Design review of the part built by this model. Coordinates are the model's own, in mm. A direction names the side the tool comes from. Round coordinates to 2 decimals unless told otherwise and drop trailing zeros. Order: outer loops, then holes, each group sorted by start corner. A loop starts at its lowest first (then second) coordinate and runs counter-clockwise, first axis right, second up. Notation, with made-up numbers: (34, -26.5) - (49, -26.5) arc R26 ccw to (49, -0.5) - close; hole circle Ø2 at (28.25, 87). An arc over 180 degrees is marked (long way). Write item = value, one per line.
from build123d import *

# Parameters (mm, degrees)
BOSS_EXTRUDE4_DEPTH = 3
FILLET1_R           = 0.5


with BuildPart() as part:
    # Sketch1 → Boss-Extrude4 (new body)
    with BuildSketch(Plane(origin=(0, 0, 0), x_dir=(1, 0, 0), z_dir=(0, 1, 0))):
        Polygon((-369.811676083, 283.948122897), (-399.811676083, 283.948122897), (-399.811676083, 243.948122897), (-319.811676083, 243.948122897), (-319.811676083, 283.948122897), (-349.811676083, 283.948122897), (-354.811676083, 283.948122897), (-354.811676083, 278.948122897), (-324.811676083, 278.948122897), (-324.811676083, 248.948122897), (-394.811676083, 248.948122897), (-394.811676083, 278.948122897), (-364.811676083, 278.948122897), (-364.811676083, 283.948122897), align=None)
        Polygon((-369.811676083, 293.948122897), (-369.811676083, 283.948122897), (-364.811676083, 283.948122897), (-364.811676083, 288.948122897), (-354.811676083, 288.948122897), (-354.811676083, 283.948122897), (-349.811676083, 283.948122897), (-349.811676083, 293.948122897), align=None)
    extrude(amount=BOSS_EXTRUDE4_DEPTH)

    # Fillet1
    fillet1_edges = [part.edges().sort_by_distance(p)[0] for p in [
        (-349.811676083, 3, -288.948122897),
        (-359.811676083, 3, -293.948122897),
        (-364.811676083, 0, -283.948122897),
        (-379.811676083, 0, -278.948122897),
        (-394.811676083, 0, -263.948122897),
        (-369.811676083, 3, -288.948122897),
        (-359.811676083, 0, -248.948122897),
        (-324.811676083, 0, -263.948122897),
        (-339.811676083, 0, -278.948122897),
        (-354.811676083, 0, -283.948122897),
        (-359.811676083, 0, -288.948122897),
        (-319.811676083, 0, -263.948122897),
        (-359.811676083, 0, -243.948122897),
        (-384.811676083, 3, -283.948122897),
        (-349.811676083, 0, -288.948122897),
        (-334.811676083, 0, -283.948122897),
        (-399.811676083, 3, -263.948122897),
        (-364.811676083, 1.5, -288.948122897),
        (-364.811676083, 1.5, -278.948122897),
        (-394.811676083, 1.5, -278.948122897),
        (-359.811676083, 3, -243.948122897),
        (-394.811676083, 1.5, -248.948122897),
        (-324.811676083, 1.5, -278.948122897),
        (-354.811676083, 1.5, -278.948122897),
        (-354.811676083, 1.5, -288.948122897),
        (-319.811676083, 1.5, -283.948122897),
        (-319.811676083, 1.5, -243.948122897),
        (-399.811676083, 1.5, -243.948122897),
        (-349.811676083, 1.5, -293.948122897),
        (-349.811676083, 1.5, -283.948122897),
        (-319.811676083, 3, -263.948122897),
        (-359.811676083, 3, -288.948122897),
        (-354.811676083, 3, -283.948122897),
        (-339.811676083, 3, -278.948122897),
        (-334.811676083, 3, -283.948122897),
        (-324.811676083, 3, -263.948122897),
        (-359.811676083, 3, -248.948122897),
        (-394.811676083, 3, -263.948122897),
        (-379.811676083, 3, -278.948122897),
        (-364.811676083, 3, -283.948122897),
    ]]
    fillet(fillet1_edges, radius=FILLET1_R)


solid = part.part
1) To check wall thickness, follow L1, parallel to X at y = 2.1, z = -263; L2, parallel to Z at x = -387, y = 1.8; L3, parallel to X at y = 2.6, z = -287.5. State the ranges of each line that lie inside material, in increasing order. Write a range as from..to.
Findings:
L1 = -399.81..-394.81, -324.81..-319.81
L2 = -283.95..-278.95, -248.95..-243.95
L3 = -369.8..-364.82, -354.8..-349.82
2) Clearance check with flat-ended pins moving along their axes: pin 1 Ø1.6 at (x, y) = (-329.5, 2) entering from -Z; pin 2 Ø0.6 at (y, z) = (2, -289) entering from +X; pin 3 Ø2 at (x, z) = (-368.5, -277) entering from -Y; pin 4 Ø0.8 at (y, z) = (2, -288) entering from -X. State where each tip first meets the part, or that it passes through.
Findings:
pin_1 = -283.95
pin_2 = -349.81
pin_3 = through
pin_4 = -369.81
3) We need section B-B on x = -352.5. Write out the cut boundary in (y, z), and give its area (3 significant figures).
Findings:
outline = (0, -293.95) - (2.5, -293.95) arc R0.5 ccw to (3, -293.45) - (3, -279.45) arc R0.5 ccw to (2.5, -278.95) - (0.5, -278.95) arc R0.5 ccw to (0, -279.45) - close; (0, -248.45) arc R0.5 ccw to (0.5, -248.95) - (2.5, -248.95) arc R0.5 ccw to (3, -248.45) - (3, -244.45) arc R0.5 ccw to (2.5, -243.95) - (0.5, -243.95) arc R0.5 ccw to (0, -244.45) - close
area = 59.6 mm^2
4) We need section A-A on z = -272.5. Write out the cut boundary in (x, y).
Findings:
outline = (-399.81, 0) - (-395.31, 0) arc R0.5 ccw to (-394.81, 0.5) - (-394.81, 2.5) arc R0.5 ccw to (-395.31, 3) - (-399.31, 3) arc R0.5 ccw to (-399.81, 2.5) - close; (-324.81, 0.5) arc R0.5 ccw to (-324.31, 0) - (-320.31, 0) arc R0.5 ccw to (-319.81, 0.5) - (-319.81, 2.5) arc R0.5 ccw to (-320.31, 3) - (-324.31, 3) arc R0.5 ccw to (-324.81, 2.5) - close
5) For faces 1 (the flat face through (-349.812, 1, -289)), 2 (the flat face through (-366, 0, -280)), 3 (the flat face through (-399.812, 1, -264)), 4 (the flat face through (-324.812, 1, -264)), 5 (the flat face through (-385, 1, -283.948)), list the 3-axis set-ups (+Z, -Z, +X, -X, +Y, -Y) from which the entire face can be reached by the end or side of a thin tool; tool diameter is ignored.
Findings:
face_1 = -Z, +X, +Y, -Y
face_2 = +Z, -Z, +X, -X, -Y
face_3 = +Z, -Z, -X, +Y, -Y
face_4 = +Y, -Y
face_5 = -Z, -X, +Y, -Y
6) The part is to be moulded in two halves that separate along Z. For faces 6 (the flat face through (-360, 1, -243.948)), 7 (the flat face through (-369.812, 1, -289)), 8 (the flat face through (-340, 1, -278.948)), say which applies: released by +Z, released by -Z, zero draft, split by the parting line, or undercut.
Findings:
face_6 = released by +Z
face_7 = zero draft
face_8 = undercut
7) We need section D-D on z = -290.5. Write out the cut boundary in (x, y), and give its area (3 significant figures).
Findings:
outline = (-369.81, 0) - (-350.31, 0) arc R0.5 ccw to (-349.81, 0.5) - (-349.81, 2.5) arc R0.5 ccw to (-350.31, 3) - (-369.31, 3) arc R0.5 ccw to (-369.81, 2.5) - close
area = 59.8 mm^2
8) We need section C-C on y = 1.3. Write out the cut boundary in (x, z), and give its area (3 significant figures).
Findings:
outline = (-399.81, -283.95) - (-369.81, -283.95) - (-369.81, -293.95) - (-350.31, -293.95) arc R0.5 ccw to (-349.81, -293.45) - (-349.81, -284.45) arc R0.5 cw to (-349.31, -283.95) - (-320.31, -283.95) arc R0.5 ccw to (-319.81, -283.45) - (-319.81, -244.45) arc R0.5 ccw to (-320.31, -243.95) - (-399.31, -243.95) arc R0.5 ccw to (-399.81, -244.45) - close; hole (-394.81, -278.45) arc R0.5 ccw to (-394.31, -278.95) - (-365.31, -278.95) arc R0.5 cw to (-364.81, -279.45) - (-364.81, -288.45) arc R0.5 ccw to (-364.31, -288.95) - (-355.31, -288.95) arc R0.5 ccw to (-354.81, -288.45) - (-354.81, -279.45) arc R0.5 cw to (-354.31, -278.95) - (-325.31, -278.95) arc R0.5 ccw to (-324.81, -278.45) - (-324.81, -248.95) - (-394.31, -248.95) arc R0.5 ccw to (-394.81, -249.45) - close
area = 1,200 mm^2
